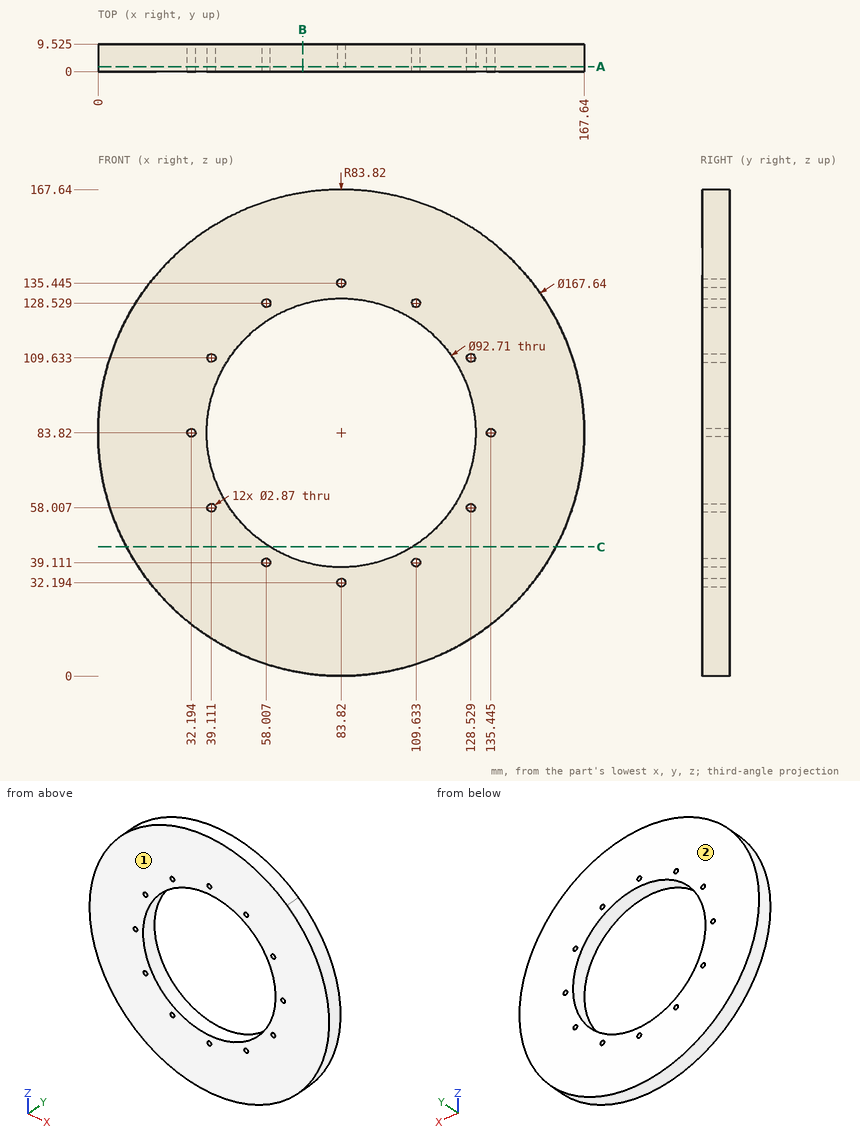
Here's the drawing with two shaded views (mm, measured from the low corner). I have some questions. Coordinates: 2 decimals unless noted, no trailing zeros. Loops run counter-clockwise (first coordinate to the right, second up) from the corner with the lowest first, then second, coordinate; pieces in that order, holes last. Notation, with made-up numbers: M 50,76.5 L 72,76.5 A10 cw 72,94.5 Z; hole C 15,-6 d6. An arc over 180 degrees is marked long. Return JSON: item names as keys, results as strings. Group by question number.
Item 1: I'm going to push flat-ended pins straight in: pin 1 Ø3 at (x, y) = (112, 1) entering from -Z; pin 2 Ø3 at (y, z) = (1.5, 109.5) entering from +X; pin 3 Ø4 at (x, y) = (78.5, 2) entering from -Z. Where does each tip first touch, or does it pass through?
Item 2: Imagine slicing it at C-C (z = 44.5). Please give me the cut outline in (x, y) (1 decimal).
Item 3: Imagine slicing it at B-B (x = 70.5). Please give me the cut outline in (y, z) (1 decimal).
Item 4: If I drill on L1, parallel to X at y = 1.25, z = 114.5 (1 decimal); L2, parallel to X at y = 2.25, z = 60 (1 decimal); L3, parallel to Z at x = 113.5, y = 8.25 (1 decimal), over which ranges is the centre line in solid material (lowest first)? Write a range as from..to.
Item 5: Imagine slicing it at A-A (y = 1.75). Give the number of separate pieces and of enclosed holes in the cut face, and give its area (3 significant figures).
Item 6: Thinking about a two-plate mould opening in Y: for the marked faces 1 and 2, which applies, released by +Y, released by -Y, zero draft, split by the parting line, or undercut?
Verdict:
{
 "1": {"pin 1": "stops at z = 4.36", "pin 2": "stops at x = 164.08", "pin 3": "stops at z = 0.07"},
 "2": {"outline": "M 9.8,0 L 59.3,0 L 59.3,9.5 L 9.8,9.5 Z; M 108.4,0 L 157.8,0 L 157.8,9.5 L 108.4,9.5 Z"},
 "3": {"outline": "M 0,1.1 L 9.5,1.1 L 9.5,39.4 L 0,39.4 Z; M 0,128.2 L 9.5,128.2 L 9.5,166.6 L 0,166.6 Z"},
 "4": {"L1": "x = 5.8..49.1, 118.6..161.8", "L2": "x = 3.5..44.1, 123.6..164.2", "L3": "z = 5.4..48.2, 119.4..162.2"},
 "5": {"separate pieces": "1", "enclosed holes": "13", "area": "15,200 mm^2"},
 "6": {"face 1": "released by -Y", "face 2": "released by +Y"}
}
